from build123d import *

# Parameters (mm, degrees)
EXTRUDE_1_DEPTH          = 220
SKETCH_3_R               = 1.55
CUT_EXTRUDE_1_DEPTH      = 10
SKETCH_4_R               = 1.55
CUT_EXTRUDE_2_DEPTH      = 120
CUT_EXTRUDE_2_DEPTH_BACK = 10


with BuildPart() as part:
    # Sketch 2 → Extrude 1 (new body)
    with BuildSketch(Plane(origin=(0, 0, 0), x_dir=(1, 0, 0), z_dir=(0, 1, 0))):
        Polygon((-87.523326774, 42.5), (-112.419250373, 17.604076401), (-112.419250373, 0), (-117.419250373, 0), (-117.419250373, 19.675144213), (-89.594394586, 47.5), (-67.523326774, 47.5), (-67.523326774, 42.5), align=None)
    extrude(amount=EXTRUDE_1_DEPTH)

    # Sketch 3 → Cut-Extrude 1 (cut)
    with BuildSketch(Plane.ZY.offset(117.419250373)):
        with Locations((-10, 5)):
            Circle(SKETCH_3_R)
        with Locations((-10, 215)):
            Circle(SKETCH_3_R)
        with Locations((-10, 110)):
            Circle(SKETCH_3_R)
    extrude(amount=-CUT_EXTRUDE_1_DEPTH, mode=Mode.SUBTRACT)

    # Sketch 4 → Cut-Extrude 2 (cut, two sides)
    with BuildSketch(Plane.XY.offset(-42.5)) as cut_extrude_2_sk:
        with Locations((-76.693326774, 5)):
            Circle(SKETCH_4_R)
        with Locations((-76.693326774, 215)):
            Circle(SKETCH_4_R)
        with Locations((-76.693326774, 110)):
            Circle(SKETCH_4_R)
    extrude(amount=CUT_EXTRUDE_2_DEPTH, mode=Mode.SUBTRACT)
    extrude(cut_extrude_2_sk.sketch, amount=-CUT_EXTRUDE_2_DEPTH_BACK, mode=Mode.SUBTRACT)


solid = part.part
Geometry check sheet. Reference: the model listing, model coordinates, mm. A direction names the side the tool comes from. Give positions to 0.01 mm unless a question says otherwise; leave off trailing zeros. Loops run counter-clockwise (first coordinate to the right, second up) from the corner with the lowest first, then second, coordinate; pieces in that order, holes last. Notation, with made-up numbers: M 3.5,62 L 20.5,62 A18 ccw 20.5,73 Z; hole C 29.25,17 d8. An arc over 180 degrees is marked long. Write each question's results on one line, items separated by ' | '.
1) Section check A-A, the plane y = 94.5. Record the boundary of the cut face in (x, z), plus the area to 3 significant figures.
Answers follow:
outline: M -117.42,-19.68 L -89.59,-47.5 L -67.52,-47.5 L -67.52,-42.5 L -87.52,-42.5 L -112.42,-17.6 L -112.42,0 L -117.42,0 Z | area: 385 mm2
2) Thickness scan on line 1 (Y direction, x = -116, z = -10); line 2 (X direction, y = 140, z = -8.5); line 3 (Z direction, x = -70, y = 40.5). Record the ranges inside material, lowest first.
Answers follow:
line 1: 0 to 3.45, 6.55 to 108.45, 111.55 to 213.45, 216.55 to 220 | line 2: -117.42 to -112.42 | line 3: -47.5 to -42.5
3) Gauge pin test, flat ends, axial feed: pin 1 (6 mm diameter, centred on x = -76.5, y = 75, fed in from +Z); pin 2 (1.9 mm diameter, centred on x = -76.69, y = 215, fed in from -Z); pin 3 (2 mm diameter, centred on y = 22.5, z = -39.5, fed in from +X); pin 4 (3.5 mm diameter, centred on y = 215, z = -10, fed in from +X). Record the tip position at first contact, or that the pin passes through.
Answers follow:
pin 1: z = -42.5 | pin 2: through | pin 3: x = -89.52 | pin 4: x = -112.42
4) Tool access check on faces 1 (the face through (-112.419, 108, -9)), 2 (the face through (-115, 108, 0)). Record the directions out of +Z, -Z, +X, -X, +Y, -Y that give a thin tool (end or side, any length) a straight path to the whole face; none if there is none.
Answers follow:
face 1: +Z, +X, +Y, -Y | face 2: +Z, +X, -X, +Y, -Y
5) Section check B-B, the plane z = -13.5. Record the boundary of the cut face in (x, y).
Answers follow:
outline: M -117.42,0 L -112.42,0 L -112.42,220 L -117.42,220 Z
6) Section check C-C, the plane x = -106.5. Record the boundary of the cut face in (y, z), plus the area to 3 significant figures.
Answers follow:
outline: M 0,-30.59 L 220,-30.59 L 220,-23.52 L 0,-23.52 Z | area: 1,560 mm2
